Here's how the part is built. I have some questions about the finished solid (model axes, mm). A direction names the side the tool comes from. Round coordinates to 2 decimals unless told otherwise and drop trailing zeros. Loops run counter-clockwise (first coordinate to the right, second up) from the corner with the lowest first, then second, coordinate; pieces in that order, holes last. Notation, with made-up numbers: M 87.25,-27.5 L 98.25,-27.5 A17 cw 98.25,-0.5 Z; hole C 73.25,58 d7. An arc over 180 degrees is marked long. Put each result on its own line as item: value. Start each with the question number.
```python
from build123d import *

# Parameters (mm, degrees)
SKETCH_1_R          = 4
EXTRUDE_1_DEPTH     = 14
SKETCH_2_R          = 2.75
CUT_EXTRUDE_1_DEPTH = 14


with BuildPart() as part:
    # 草图1 → 凸台-拉伸1 (new body)
    with BuildSketch(Plane.XY):
        Polygon((-21, -10.75), (-9, -10.75), (-9, 16.25), (9, 16.25), (9, -10.75), (21, -10.75), (21, -16.25), (-21, -16.25), align=None)
        with Locations((0, 3.75)):
            Circle(SKETCH_1_R, mode=Mode.SUBTRACT)
    extrude(amount=EXTRUDE_1_DEPTH)

    # 草图2 → 切除-拉伸1 (cut)
    with BuildSketch(Plane(origin=(0, -10.75, 0), x_dir=(1, 0, 0), z_dir=(0, 1, 0))):
        with Locations(Location((-16.25, -7, 0), (0, 0, 270))):
            Circle(SKETCH_2_R)
        with Locations(Location((16.25, -7, 0), (0, 0, 270))):
            Circle(SKETCH_2_R)
    extrude(amount=-CUT_EXTRUDE_1_DEPTH, mode=Mode.SUBTRACT)


solid = part.part
```
1) If we mould it in two halves opening along Z, with no side actions, what happens to faces 4 (the face through (0, -3, 14)), 5 (the face through (-9, 3, 7)), 6 (the face through (-13.93, -13.46, 8.48))? For each: pulls with the +Z half, pulls with the -Z half, needs draft (parallel to the pull), parting line crosses it, or undercut.
2) Suppose I cut it at A-A (z = 7). Write out the boundary of the cut face in (x, y), plus the area to 3 significant figures.
3) Suppose I cut it at D-D (z = 12.75). Write out the boundary of the cut face in (x, y), plus the area to 3 significant figures.
4) Suppose I cut it at C-C (y = 3.75). Write out the boundary of the cut face in (x, z).
5) I'm going to push flat-ended pins straight in: P1, Ø5, axis at y = 11.5, z = 3, coming from the -X side; P2, Ø3.5, axis at x = -16.25, z = 7, coming from the +Y side. Where does each tip first touch, or does it pass through?
6) If I drill on probe 1 along X at (y, z) = (-12, 7); probe 2 along X at (y, z) = (4, 12.75); probe 3 along Z at (x, y) = (16, -13), over which ranges is the centre line in solid material (lowest first)? Write a range as from..to.
7) Suppose I cut it at B-B (x = 0). Write out the boundary of the cut face in (y, z).
8) On a 3-axis mill with a long thin cutter (end or side, diameter ignored), from which of +Z, -Z, +X, -X, +Y, -Y can I reach the whole of each face in a straight line? I mean faces 1 (the face through (-14, -10.75, 5)), 2 (the face through (13.6, -10.75, 8.5)), 3 (the face through (0, -16.25, 7)). Say none if no direction works.
Results are:
1. face 4: pulls with the +Z half
1. face 5: needs draft
1. face 6: undercut
2. outline: M -21,-16.25 L -19,-16.25 L -19,-10.75 L -21,-10.75 Z; M -13.5,-16.25 L 13.5,-16.25 L 13.5,-10.75 L 9,-10.75 L 9,16.25 L -9,16.25 L -9,-10.75 L -13.5,-10.75 Z; M 19,-16.25 L 21,-16.25 L 21,-10.75 L 19,-10.75 Z; hole C 0,3.75 d8
2. area: 606 mm²
3. outline: M -21,-16.25 L 21,-16.25 L 21,-10.75 L 9,-10.75 L 9,16.25 L -9,16.25 L -9,-10.75 L -21,-10.75 Z; hole C 0,3.75 d8
3. area: 667 mm²
4. outline: M -9,0 L -4,0 L -4,14 L -9,14 Z; M 4,0 L 9,0 L 9,14 L 4,14 Z
5. P1: x = -9
5. P2: through
6. probe 1: -21..-19, -13.5..13.5, 19..21
6. probe 2: -9..-3.99, 3.99..9
6. probe 3: 0..4.26, 9.74..14
7. outline: M -16.25,0 L -0.25,0 L -0.25,14 L -16.25,14 Z; M 7.75,0 L 16.25,0 L 16.25,14 L 7.75,14 Z
8. face 1: +Z, -Z, -X, +Y
8. face 2: +Z, -Z, +X, +Y
8. face 3: +Z, -Z, +X, -X, -Y
